```python
from build123d import *

# Parameters (mm, degrees)
SKETCH_1_R          = 6
EXTRUDE_1_DEPTH     = 5
SKETCH_3_R          = 4
EXTRUDE_2_DEPTH     = 5
EXTRUDE_3_DEPTH     = 5
SKETCH_2_R          = 5
CUT_EXTRUDE_1_DEPTH = 6
SKETCH_5_R          = 4
EXTRUDE_4_DEPTH     = 12
SKETCH_6_W          = 10.625447748
SKETCH_6_H          = 3
CUT_EXTRUDE_2_DEPTH = 18


with BuildPart() as part:
    # Sketch 1 → Extrude 1 (new body)
    with BuildSketch(Plane(origin=(0, 0, 0), x_dir=(1, 0, 0), z_dir=(0, 1, 0))):
        Circle(SKETCH_1_R)
    extrude(amount=EXTRUDE_1_DEPTH)



with BuildPart() as body_2:
    # Sketch 3 → Extrude 2 (new body)
    with BuildSketch(Plane(origin=(0, 0, 0), x_dir=(1, 0, 0), z_dir=(0, 1, 0))):
        with Locations((10.373073214, 0)):
            Circle(SKETCH_3_R)
    extrude(amount=EXTRUDE_2_DEPTH)


with BuildPart() as part_1:
    add(part.part)

    add(body_2.part)  # Extrude 3 merges body 2
    # Sketch 4 → Extrude 3 (add)
    with BuildSketch(Plane(origin=(0, 0, 0), x_dir=(1, 0, 0), z_dir=(0, 1, 0))):
        Polygon((0, 6), (10.373073214, 4), (10.373073214, -4), (0, -6), align=None)
    extrude(amount=EXTRUDE_3_DEPTH)

    # Sketch 2 → Cut-Extrude 1 (cut, through all)
    with BuildSketch(Plane(origin=(0, 5, 0), x_dir=(1, 0, 0), z_dir=(0, 1, 0))):
        Circle(SKETCH_2_R)
    extrude(amount=-CUT_EXTRUDE_1_DEPTH, mode=Mode.SUBTRACT)

    # Sketch 5 → Extrude 4 (add)
    with BuildSketch(Plane(origin=(0, 5, 0), x_dir=(1, 0, 0), z_dir=(0, 1, 0))):
        with Locations((10.373073214, 0)):
            Circle(SKETCH_5_R)
    extrude(amount=EXTRUDE_4_DEPTH)

    # Sketch 6 → Cut-Extrude 2 (cut, through all)
    with BuildSketch(Plane(origin=(0, 17, 0), x_dir=(1, 0, 0), z_dir=(0, 1, 0))):
        with Locations((13.66467232, 0)):
            Rectangle(SKETCH_6_W, SKETCH_6_H)
    extrude(amount=-CUT_EXTRUDE_2_DEPTH, mode=Mode.SUBTRACT)


solid = part_1.part
```
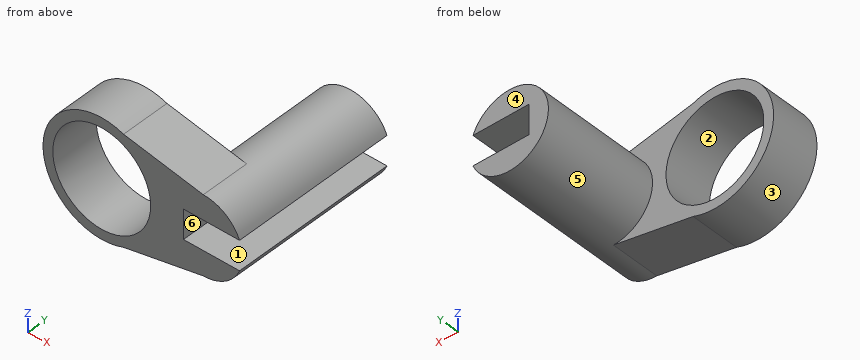
Work out the finished part from the listing and answer in its coordinate system (mm). Face numbers are marked on the shaded views. A direction names the side the tool comes from. Round coordinates to 2 decimals unless told otherwise and drop trailing zeros. Order: outer loops, then holes, each group sorted by start corner. A loop starts at its lowest first (then second) coordinate and runs counter-clockwise, first axis right, second up.
Q1. Given pin 1 Ø4 at (x, z) = (11, 0) entering from -Y; pin 2 Ø5 at (y, z) = (10.5, -4.5) entering from -X; pin 3 Ø1.7 at (x, y) = (10.5, 5.5) entering from -Z; pin 4 Ø1 at (y, z) = (3.5, -1) entering from -X, each flat-ended and moving along its own axis, determine where each tip first touches the part or whether it passes through.
Solution:
pin 1: stops at y = 0
pin 2: stops at x = 6.91
pin 3: stops at z = -4.11
pin 4: stops at x = -5.98
Q2. A tool of negligible diameter and unlimited length cuts with its end or side. For the marked faces 4, 5 and 6, from which of +Z, -Z, +X, -X, +Y, -Y can it reach the whole face along a straight path? Write none if from no direction.
Solution:
face 4: +Z, -Z, +X, -X, +Y
face 5: +Y
face 6: +X, +Y, -Y
Q3. A cutting plane is placed at B-B, the plane x = 0. Determine the outline of the cut face in (y, z), then the cut area to 3 significant figures.
Solution:
outline: (0, -6) - (5, -6) - (5, -5) - (0, -5) - close; (0, 5) - (5, 5) - (5, 6) - (0, 6) - close
area: 10.0 mm2
Q4. Find the intervals of material crossed by line 1 along X through (y, z) = (2.9, 0); line 2 along Z through (x, y) = (0, 2.2); line 3 along Z through (x, y) = (10.5, 5.5), in increasing order.
Solution:
line 1: x = -6 to -5, 5 to 8.35
line 2: z = -6 to -5, 5 to 6
line 3: z = -4 to -1.5, 1.5 to 4
Q5. A cutting plane is placed at A-A, the plane z = 0. Determine the outline of the cut face in (x, y).
Solution:
outline: (-6, 0) - (-5, 0) - (-5, 5) - (-6, 5) - close; (5, 0) - (8.35, 0) - (8.35, 17) - (6.37, 17) - (6.37, 5) - (5, 5) - close
Q6. The mould has two halves that part along X. Classify the marked faces 1, 2 and 3: pulls with the +X half, pulls with the -X half, needs draft (parallel to the pull), parting line crosses it, or undercut.
Solution:
face 1: needs draft
face 2: undercut
face 3: parting line crosses it
Q7. A cutting plane is placed at C-C, the plane y = 4.5. Determine the outline of the cut face in (x, z), then the cut area to 3 significant figures.
Solution:
outline: (2.23, -5.57) - (10.37, -4) arc R4 ccw to (14.08, -1.5) - (8.35, -1.5) - (8.35, 1.5) - (14.08, 1.5) arc R4 ccw to (10.37, 4) - (2.23, 5.57) arc R6 ccw (long way) to start; hole circle Ø10 at (0, 0)
area: 89.4 mm2
Q8. A cutting plane is placed at D-D, the plane z = -2.25. Determine the outline of the cut face in (x, y).
Solution:
outline: (-5.56, 0) - (-4.47, 0) - (-4.47, 5) - (-5.56, 5) - close; (4.47, 0) - (13.68, 0) - (13.68, 17) - (7.07, 17) - (7.07, 5) - (4.47, 5) - close
